```python
from build123d import *

# Parameters (mm, degrees)
SKETCH1_R           = 28.5
SKETCH1_R_2         = 2.5
BOSS_EXTRUDE1_DEPTH = 17.5
SKETCH2_R           = 9
CUT_EXTRUDE1_DEPTH  = 18.5
CHAMFER1_SIZE       = 2


with BuildPart() as part:
    # Sketch1 → Boss-Extrude1 (new body)
    with BuildSketch(Plane.XY):
        Circle(SKETCH1_R)
        with Locations((0, 23.75)):
            Circle(SKETCH1_R_2, mode=Mode.SUBTRACT)
        with Locations((20.56810334, 11.875)):
            Circle(SKETCH1_R_2, mode=Mode.SUBTRACT)
        with Locations((20.56810334, -11.875)):
            Circle(SKETCH1_R_2, mode=Mode.SUBTRACT)
        with Locations((0, -23.75)):
            Circle(SKETCH1_R_2, mode=Mode.SUBTRACT)
        with Locations((-20.56810334, -11.875)):
            Circle(SKETCH1_R_2, mode=Mode.SUBTRACT)
        with Locations((-20.56810334, 11.875)):
            Circle(SKETCH1_R_2, mode=Mode.SUBTRACT)
    extrude(amount=BOSS_EXTRUDE1_DEPTH)

    # Sketch2 → Cut-Extrude1 (cut, through all)
    with BuildSketch(Plane.XY.offset(17.5)):
        Circle(SKETCH2_R)
    extrude(amount=-CUT_EXTRUDE1_DEPTH, mode=Mode.SUBTRACT)

    # Chamfer1
    chamfer1_edges = [part.edges().sort_by_distance(p)[0] for p in [
        (-9, 0, 0),
        (-9, 0, 17.5),
    ]]
    chamfer(chamfer1_edges, length=CHAMFER1_SIZE)


solid = part.part
```
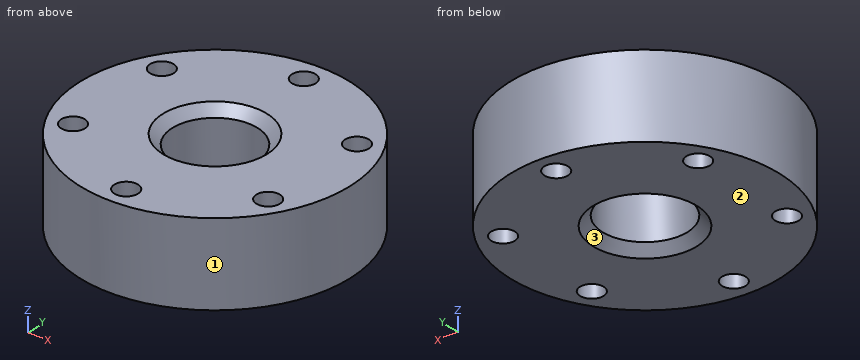
Input: part model. Units: mm. Frame: model coordinates. Face numbers are marked on the shaded views. Coordinates: 2 decimals unless noted, no trailing zeros. Loops run counter-clockwise (first coordinate to the right, second up) from the corner with the lowest first, then second, coordinate; pieces in that order, holes last. Notation, with made-up numbers: M 59.5,11.25 L 86.5,11.25 A14 ccw 86.5,33.25 Z; hole C 78.5,-1.75 d9. An arc over 180 degrees is marked long. One line per item, written item: value.
(1) Pin query (flat end, axial travel): pin 1 (1 mm diameter, centred on x = -9, z = 15.5, fed in from -Y); pin 2 (2 mm diameter, centred on x = 11, z = 2, fed in from -Y); pin 3 (2 mm diameter, centred on y = -6.5, z = 4.5, fed in from +X). Return the tip coordinate at first contact, or that it passes through.
Filled in:
pin 1: y = -27.2
pin 2: y = -26.69
pin 3: x = 27.96
(2) Section B-B (x = 0). Output: boundary loops of the cut face in (y, z).
Filled in:
outline: M -28.5,0 L -26.25,0 L -26.25,17.5 L -28.5,17.5 Z; M -21.25,0 L -11,0 L -9,2 L -9,15.5 L -11,17.5 L -21.25,17.5 Z; M 9,2 L 11,0 L 21.25,0 L 21.25,17.5 L 11,17.5 L 9,15.5 Z; M 26.25,0 L 28.5,0 L 28.5,17.5 L 26.25,17.5 Z
(3) Section D-D (z = 11). Output: boundary loops of the cut face in (x, y) (3 decimals).
Filled in:
outline: C 0,0 d57; hole C -20.568,-11.875 d5; hole C -20.568,11.875 d5; hole C 0,0 d18; hole C 0,-23.75 d5; hole C 0,23.75 d5; hole C 20.568,-11.875 d5; hole C 20.568,11.875 d5
(4) Line query: line 1 along Y through (x, z) = (0, 8.25); line 2 along Y through (x, z) = (-19, 9.75); line 3 along X through (y, z) = (13.5, 15.5). Output: solid intervals per line, ascending. Write a range as from..to.
Filled in:
line 1: -28.5..-26.25, -21.25..-9, 9..21.25, 26.25..28.5
line 2: -21.24..-13.82, -9.93..9.93, 13.82..21.24
line 3: -25.1..-22.47, -18.67..18.67, 22.47..25.1
(5) Pull-direction query (X, two-part tool) for the marked faces 1, 2 and 3; classes: +X half, -X half, draft (parallel to the pull), parting line (faces both ways), or undercut.
Filled in:
face 1: parting line
face 2: draft
face 3: undercut
(6) Section C-C (x = 22). Output: boundary loops of the cut face in (y, z), and give its area (3 significant figures).
Filled in:
outline: M -18.12,0 L -13.92,0 L -13.92,17.5 L -18.12,17.5 Z; M -9.83,0 L 9.83,0 L 9.83,17.5 L -9.83,17.5 Z; M 13.92,0 L 18.12,0 L 18.12,17.5 L 13.92,17.5 Z
area: 491 mm^2
(7) Section A-A (y = 0). Output: boundary loops of the cut face in (x, z), and give its area (4 significant figures).
Filled in:
outline: M -28.5,0 L -11,0 L -9,2 L -9,15.5 L -11,17.5 L -28.5,17.5 Z; M 9,2 L 11,0 L 28.5,0 L 28.5,17.5 L 11,17.5 L 9,15.5 Z
area: 674.5 mm^2
